```python
from build123d import *

# Parameters (mm, degrees)
SKETCH1_W                                           = 19.939
SKETCH1_H                                           = 24.2062
BOSS_EXTRUDE1_DEPTH                                 = 6.604
F_4_40_TAPPED_HOLE1_D                               = 2.2606
F_4_40_TAPPED_HOLE1_DEPTH                           = 6.604
CBORE_FOR_4_BINDING_HEAD_MACHINE_SCREW3_D           = 3.2639
CBORE_FOR_4_BINDING_HEAD_MACHINE_SCREW3_CBORE_D     = 4.9022
CBORE_FOR_4_BINDING_HEAD_MACHINE_SCREW3_CBORE_DEPTH = 1.7272
FILLET1_R                                           = 6.35
FILLET2_R                                           = 3.175


with BuildPart() as part:
    # Sketch1 → Boss-Extrude1 (new body)
    with BuildSketch(Plane(origin=(0, 0, 0), x_dir=(1, 0, 0), z_dir=(0, 1, 0))):
        with Locations((0, 12.1031)):
            Rectangle(SKETCH1_W, SKETCH1_H)
    extrude(amount=BOSS_EXTRUDE1_DEPTH)

    # #4-40 Tapped Hole1
    with Locations(Plane(origin=(0, 6.604, 0), x_dir=(1, 0, 0), z_dir=(0, 1, 0))):
        with Locations((3.81, 16.129), (3.81, 6.731)):
            Hole(F_4_40_TAPPED_HOLE1_D / 2, depth=F_4_40_TAPPED_HOLE1_DEPTH)

    # CBORE for #4 Binding Head Machine Screw3 (through all)
    with Locations(Plane(origin=(0, 0, 0), x_dir=(-1, 0, 0), z_dir=(0, -1, 0))):
        with Locations((6.35, 3.8862), (-6.35, 3.8862)):
            CounterBoreHole(CBORE_FOR_4_BINDING_HEAD_MACHINE_SCREW3_D / 2, CBORE_FOR_4_BINDING_HEAD_MACHINE_SCREW3_CBORE_D / 2, CBORE_FOR_4_BINDING_HEAD_MACHINE_SCREW3_CBORE_DEPTH)

    # Fillet1
    fillet1_edges = [part.edges().sort_by_distance(p)[0] for p in [
        (9.9695, 3.302, -24.2062),
    ]]
    fillet(fillet1_edges, radius=FILLET1_R)

    # Fillet2
    fillet2_edges = [part.edges().sort_by_distance(p)[0] for p in [
        (-9.9695, 3.302, -24.2062),
    ]]
    fillet(fillet2_edges, radius=FILLET2_R)


solid = part.part
```
Here's how the part is built. I have some questions about the finished solid (model axes, mm). A direction names the side the tool comes from. Coordinates: 2 decimals unless noted, no trailing zeros. Order: outer loops, then holes, each group sorted by start corner. A loop starts at its lowest first (then second) coordinate and runs counter-clockwise, first axis right, second up.
Item 1: I'm going to push a flat-ended pin straight in: pin 1 Ø4.5 at (x, z) = (-6.35, -3.89) entering from -Y. Where does the tip first touch, or does it pass through?
Response values:
pin 1: stops at y = 1.73
Item 2: If we section it at A-A, the plane x = -6.35: List the corners of the cut face in (y, z) for me, then the cut area to 3 significant figures.
Response values:
outline: (0, -24.21) - (6.6, -24.21) - (6.6, -5.52) - (1.73, -5.52) - (1.73, -6.34) - (0, -6.34) - close; (0, -1.44) - (1.73, -1.44) - (1.73, -2.25) - (6.6, -2.25) - (6.6, 0) - (0, 0) - close
area: 135 mm2
Item 3: Thinking about a two-plate mould opening in Z: for faces 3 (the face through (8.06, 3.348, -22.395)), 4 (the face through (0, 0, -12)), 5 (the face through (-7.55, 4.2, -4.99)), 6 (the face through (4.72, 4.2, -3.96)), which applies, pulls with the +Z half, pulls with the -Z half, needs draft (parallel to the pull), parting line crosses it, or undercut?
Response values:
face 3: pulls with the -Z half
face 4: needs draft
face 5: undercut
face 6: undercut
Item 4: Which directions (+Z, -Z, +X, -X, +Y, -Y) give clear straight access to the entire face, cutting with the end or side of a thin tool? Please do faces 1 (the face through (-7.48, 0.85, -1.71)), 2 (the face through (4.055, 3.256, -15.026)).
Response values:
face 1: -Y
face 2: +Y, -Y
Item 5: I need wall thicknesses on probe 1 along Z at (x, y) = (3.81, 3.75); probe 2 along Z at (x, y) = (3.25, 3.75); probe 3 along Y at (x, z) = (5, -5.75). Which ranges of each line are inside material? Lowest first, please.
Response values:
probe 1: z = -24.2 to -17.26, -15 to -7.86, -5.6 to 0
probe 2: z = -24.21 to -17.11, -15.15 to -7.71, -5.75 to 0
probe 3: y = 1.73 to 6.6
Item 6: If we section it at C-C, the plane y = 3.5: Give the number of separate pieces and of enclosed holes in the cut face, then the cut area to 3 significant figures.
Response values:
separate pieces: 1
enclosed holes: 4
area: 447 mm2
Item 7: If we section it at B-B, the plane z = -3: List the corners of the cut face in (x, y) for me, then the cut area to 3 significant figures.
Response values:
outline: (-9.97, 0) - (-8.64, 0) - (-8.64, 1.73) - (-7.72, 1.73) - (-7.72, 6.6) - (-9.97, 6.6) - close; (-4.98, 1.73) - (-4.06, 1.73) - (-4.06, 0) - (4.06, 0) - (4.06, 1.73) - (4.98, 1.73) - (4.98, 6.6) - (-4.98, 6.6) - close; (7.72, 1.73) - (8.64, 1.73) - (8.64, 0) - (9.97, 0) - (9.97, 6.6) - (7.72, 6.6) - close
area: 89.2 mm2
Item 8: If we section it at D-D, the plane z = -15.5: List the corners of the cut face in (x, y) for me.
Response values:
outline: (-9.97, 0) - (2.87, 0) - (2.87, 6.6) - (-9.97, 6.6) - close; (4.75, 0) - (9.97, 0) - (9.97, 6.6) - (4.75, 6.6) - close
